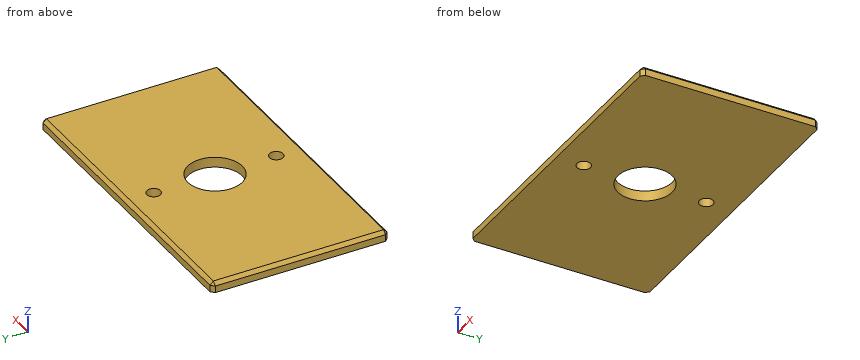
from build123d import *

# Parameters (mm, degrees)
SKETCH1_W           = 45
SKETCH1_H           = 26
SKETCH1_R           = 4
SKETCH1_R_2         = 1
BOSS_EXTRUDE1_DEPTH = 0.75
CHAMFER1_SIZE       = 0.5


with BuildPart() as part:
    # Sketch1 → Boss-Extrude1 (new body, symmetric)
    with BuildSketch(Plane.XY):
        Rectangle(SKETCH1_W, SKETCH1_H)
        Circle(SKETCH1_R, mode=Mode.SUBTRACT)
        with Locations((0, 9)):
            Circle(SKETCH1_R_2, mode=Mode.SUBTRACT)
        with Locations((0, -9)):
            Circle(SKETCH1_R_2, mode=Mode.SUBTRACT)
    extrude(amount=BOSS_EXTRUDE1_DEPTH, both=True)

    # Chamfer1
    chamfer1_edges = [part.edges().sort_by_distance(p)[0] for p in [
        (-22.5, 0, 0.75),
        (0, -13, 0.75),
        (22.5, 0, 0.75),
        (22.5, -13, 0),
        (-22.5, -13, 0),
        (-22.5, 13, 0),
        (22.5, 13, 0),
        (0, 13, 0.75),
    ]]
    chamfer(chamfer1_edges, length=CHAMFER1_SIZE)


solid = part.part
The listing builds one solid part. Answer for the finished solid, in the listing's coordinates (mm). Round coordinates to 2 decimals unless told otherwise and drop trailing zeros. Order: outer loops, then holes, each group sorted by start corner. A loop starts at its lowest first (then second) coordinate and runs counter-clockwise, first axis right, second up. Notation, with made-up numbers: (-2, -21) -> (20, -21) arc R11 cw to (20, -5) -> close; hole circle Ø9 at (75.25, -22.75). An arc over 180 degrees is marked (long way). One line per item, written item: value.
Item 1: Find section C-C, the plane z = -0.25. Give the vertices of the cut face in (x, y), then the cut area to 3 significant figures.
Taken from the geometry:
outline: (-22.5, -12.5) -> (-22, -13) -> (22, -13) -> (22.5, -12.5) -> (22.5, 12.5) -> (22, 13) -> (-22, 13) -> (-22.5, 12.5) -> close; hole circle Ø8 at (0, 0); hole circle Ø2 at (0, -9); hole circle Ø2 at (0, 9)
area: 1,110 mm2
Item 2: Find section B-B, the plane y = 0. Give the vertices of the cut face in (x, z).
Taken from the geometry:
outline: (-22.5, -0.75) -> (-4, -0.75) -> (-4, 0.75) -> (-22, 0.75) -> (-22.5, 0.25) -> close; (4, -0.75) -> (22.5, -0.75) -> (22.5, 0.25) -> (22, 0.75) -> (4, 0.75) -> close
Item 3: Find section A-A, the plane x = 0. Give the vertices of the cut face in (y, z).
Taken from the geometry:
outline: (-13, -0.75) -> (-10, -0.75) -> (-10, 0.75) -> (-12.5, 0.75) -> (-13, 0.25) -> close; (-8, -0.75) -> (-4, -0.75) -> (-4, 0.75) -> (-8, 0.75) -> close; (4, -0.75) -> (8, -0.75) -> (8, 0.75) -> (4, 0.75) -> close; (10, -0.75) -> (13, -0.75) -> (13, 0.25) -> (12.5, 0.75) -> (10, 0.75) -> close
Item 4: Straight lines are drawn through the part: L1, parallel to Y at x = 0, z = -0.25; L2, parallel to Y at x = -2, z = -0.7; L3, parallel to Y at x = 1.5, z = -0.1. For each, find the intervals that lie inside material, in ascending order.
Taken from the geometry:
L1: y = -13 to -10, -8 to -4, 4 to 8, 10 to 13
L2: y = -13 to -3.46, 3.46 to 13
L3: y = -13 to -3.71, 3.71 to 13
